from build123d import *

# Parameters (mm, degrees)
SKETCH1_W     = 88.9
SKETCH1_H     = 5
CHAMFER1_SIZE = 0.4
TAP4_D        = 4.134
TAP4_DEPTH    = 12.4
TAP4_TIP      = 1.2419789
TAP5_D        = 4.134
TAP5_DEPTH    = 12.4
TAP5_TIP      = 1.2419789


with BuildPart() as part:
    # Sketch1 → Revolve1 (revolve)
    with BuildSketch(Plane.XY):
        with Locations((44.45, 2.5)):
            Rectangle(SKETCH1_W, SKETCH1_H)
    revolve(axis=Axis((0, 0, 0), (1, 0, 0)))

    # Chamfer1
    chamfer1_edges = [part.edges().sort_by_distance(p)[0] for p in [
        (0, -5, 0),
        (88.9, -5, 0),
    ]]
    chamfer(chamfer1_edges, length=CHAMFER1_SIZE)

    # Tap4
    with Locations(Plane.ZY):
        with Locations((0, 0)):
            Hole(TAP4_D / 2, depth=TAP4_DEPTH)
            with Locations((0, 0, -(TAP4_DEPTH + TAP4_TIP / 2))):  # 118° drill point
                Cone(0, TAP4_D / 2, TAP4_TIP, mode=Mode.SUBTRACT)

    # Tap5
    with Locations(Plane(origin=(88.9, 0, 0), x_dir=(0, 0, -1), z_dir=(1, 0, 0))):
        with Locations((0, 0)):
            Hole(TAP5_D / 2, depth=TAP5_DEPTH)
            with Locations((0, 0, -(TAP5_DEPTH + TAP5_TIP / 2))):  # 118° drill point
                Cone(0, TAP5_D / 2, TAP5_TIP, mode=Mode.SUBTRACT)


solid = part.part
The listing builds one solid part. Answer for the finished solid, in the listing's coordinates (mm). A direction names the side the tool comes from. Give positions to 0.01 mm unless a question says otherwise; leave off trailing zeros. Write each loop counter-clockwise with the first axis right and the second up, starting at its lowest first coordinate (ties: lowest second). Pieces come first, ordered by that corner, then holes. Notation, with made-up numbers: (44, 19) -> (64, 19) arc R17 cw to (64, 39) -> close; hole circle Ø5 at (19, 4). An arc over 180 degrees is marked (long way). Use a Markdown table: item, result.
(1) Determine the mould class of faces 1 (the cylindrical face through (45.07, -1.08, -4.88)), 2 (the conical face through (13.426, -0.35, -0.078)), 3 (the flat face through (0, -1, -2)), 4 (the cylindrical face through (82.61, -1.26, -1.64)) for opening direction Z: released by +Z, released by -Z, zero draft, split by the parting line, or undercut.
Return value:
| item | result |
|---|---|
| face 1 | split by the parting line |
| face 2 | undercut |
| face 3 | zero draft |
| face 4 | undercut |
(2) For faces 5 (the cylindrical face through (6.29, -1.26, 1.64)), 6 (the flat face through (88.9, -1, -2)), determine the directions among +Z, -Z, +X, -X, +Y, -Y from which every point of the face is accessible in a straight line to the end or side of a thin tool.
Return value:
| item | result |
|---|---|
| face 5 | -X |
| face 6 | +Z, -Z, +X, +Y, -Y |
(3) Find the intervals of material crossed by probe 1 along Z at (x, y) = (3.75, 0); probe 2 along Z at (x, y) = (24, 2); probe 3 along Z at (x, y) = (71.5, -0.25), in increasing order. Write a range as from..to.
Return value:
| item | result |
|---|---|
| probe 1 | -5..-2.07, 2.07..5 |
| probe 2 | -4.58..4.58 |
| probe 3 | -4.99..4.99 |
(4) Flat-ended cylindrical pins translate along their axes: P1, Ø1, axis at y = 1, z = 0.5, coming from the -X side; P2, Ø5.5, axis at y = 0, z = 0, coming from the +X side. Find the tip coordinate at first contact, or state that the pin passes through.
Return value:
| item | result |
|---|---|
| P1 | x = 12.67 |
| P2 | x = 88.9 |
(5) Section A-A, the plane x = 33 is taken. Determine the outline of the cut face in (y, z).
Return value:
| item | result |
|---|---|
| outline | circle Ø10 at (0, 0) |
